Autodesk Fusion 360 part; units mm, degrees
sketch "Sketch1" plane through (0, 0, 0) normal (0, 1, 0) x (1, 0, 0)
  line L0 (125, 125) -> (-125, 125) construction
  line L1 (-125, 125) -> (-125, -125) construction
  line L2 (-125, -125) -> (125, -125) construction
  line L3 (125, -125) -> (125, 125) construction
  line L4 (125, 125) -> (-125, -125) construction
  line L5 (-125, 125) -> (125, -125) construction
  line L6 (75, 112.1152) -> (-75, 112.1152) construction
  line L7 (-75, 112.1152) -> (-75, 91.9152) construction
  line L8 (-75, 91.9152) -> (75, 91.9152) construction
  line L9 (75, 91.9152) -> (75, 112.1152) construction
  line L10 (75, 112.1152) -> (-75, 91.9152) construction
  line L11 (-75, 112.1152) -> (75, 91.9152) construction
  line L12 (137, 137) -> (92, 137)
  line L13 (92, 137) -> (137, 92)
  line L14 (137, 92) -> (137, 137)
  line L15 (125, 125) -> (137, 137) construction
  line L16 (128, 128) -> (109, 128) construction
  line L17 (109, 128) -> (128, 109) construction
  line L18 (128, 109) -> (128, 128) construction
  line L19 (92, 137) -> (84, 137)
  line L20 (84, 137) -> (84, 114)
  line L21 (84, 114) -> (104, 114)
  line L22 (104, 114) -> (114, 104)
  line L23 (114, 104) -> (114, 84)
  line L24 (114, 84) -> (137, 84)
  line L25 (137, 84) -> (137, 92)
  line L26 (84, 138) -> (-84, 138)
  line L27 (-84, 138) -> (-84, 113)
  line L28 (-84, 113) -> (84, 113)
  line L29 (84, 113) -> (84, 138)
  line L30 (84, 138) -> (-84, 113) construction
  line L31 (-84, 138) -> (84, 113) construction
  point P0 (0, 102.0152)
  point P1 (0, 125.5)
  dimension "d4" = 250
  dimension "d5" = 250
  dimension "d6" = 150
  dimension "d7" = 20.2
  dimension "d8" = 12
  dimension "d9" = 12
  dimension "d10" = 45
  dimension "d11" = 16
  dimension "d12" = 3
  dimension "d13" = 8
  dimension "d14" = 23
  dimension "d15" = 20
  dimension "d16" = 25
  dimension "d17" = 1
ref_plane "WorkPlane1" through (0, 7, 0) normal (0, 1, 0) x (0, 0, 1)
extrude "Extrude1" add sketch "Sketch1" along normal blind 4 contours L20 L26 L27 L28 L29
sketch "Sketch6" plane through (0, 4, 0) normal (0, 1, 0) x (-1, 0, 0)
  line L0 (-84, -113) -> (-84, -138)
  line L1 (-84, -138) -> (84, -138)
  line L2 (84, -138) -> (84, -113)
  line L3 (84, -113) -> (-84, -113)
  line L4 (-75, -135.575) -> (75, -135.575)
  line L5 (75, -135.575) -> (75, -115.425)
  line L6 (75, -115.425) -> (-75, -115.425)
  line L7 (-75, -115.425) -> (-75, -135.575)
  line L8 (-75, -135.575) -> (75, -115.425) construction
  line L9 (75, -135.575) -> (-75, -115.425) construction
  point P0 (0, -125.5)
  point P1 (0, -113)
  point P2 (84, -125.5)
  dimension "d36" = 150
  dimension "d37" = 20.15
extrude "Extrude4" add sketch "Sketch6" along normal up to surface (3 mm away) contours L4 L5 L6 L7
sketch "Sketch7" plane through (0, 4, 0) normal (0, 1, 0) x (-1, 0, 0)
  line L0 (75, -135.575) -> (-75, -135.575)
  line L1 (-75, -135.575) -> (-75, -115.425)
  line L2 (-75, -115.425) -> (75, -115.425)
  line L3 (75, -115.425) -> (75, -135.575)
  line L4 (-84, -113) -> (-84, -138)
  line L5 (-84, -138) -> (84, -138)
  line L6 (84, -138) -> (84, -113)
  line L7 (84, -113) -> (-84, -113)
  line L8 (-5, -135.575) -> (5, -135.575)
  line L9 (5, -135.575) -> (5, -138)
  line L10 (5, -138) -> (-5, -138)
  line L11 (-5, -138) -> (-5, -135.575)
  line L12 (-5, -135.575) -> (5, -138) construction
  line L13 (5, -135.575) -> (-5, -138) construction
  line L14 (-5, -113) -> (5, -113)
  line L15 (5, -113) -> (5, -115.425)
  line L16 (5, -115.425) -> (-5, -115.425)
  line L17 (-5, -115.425) -> (-5, -113)
  line L18 (-5, -113) -> (5, -115.425) construction
  line L19 (5, -113) -> (-5, -115.425) construction
  line L20 (-75, -135.575) -> (-65, -135.575)
  line L21 (-65, -135.575) -> (-65, -138)
  line L22 (-65, -138) -> (-75, -138)
  line L23 (-75, -138) -> (-75, -135.575)
  line L24 (-75, -115.425) -> (-65, -115.425)
  line L25 (-65, -115.425) -> (-65, -113)
  line L26 (-65, -113) -> (-75, -113)
  line L27 (-75, -113) -> (-75, -115.425)
  line L28 (75, -135.575) -> (65, -135.575)
  line L29 (65, -135.575) -> (65, -138)
  line L30 (65, -138) -> (75, -138)
  line L31 (75, -138) -> (75, -135.575)
  line L32 (75, -115.425) -> (65, -115.425)
  line L33 (65, -115.425) -> (65, -113)
  line L34 (65, -113) -> (75, -113)
  line L35 (75, -113) -> (75, -115.425)
  point P0 (0, -136.7875)
  point P1 (0, -114.2125)
  dimension "d42" = 10
extrude "Extrude5" add sketch "Sketch7" along normal blind 8 contours L0 L5 L28 L29 L30 L31 | L2 L7 L32 L33 L34 L35 | L0 L5 L8 L9 L10 L11 | L2 L7 L14 L15 L16 L17 | L0 L5 L20 L21 L22 L23 | L2 L7 L24 L25 L26 L27
chamfer "Chamfer1" distance 2 angle 45 12 edges at (-5, 12, -136.7875) (5, 12, -136.7875) (-5, 12, -114.2125) (5, 12, -114.2125) (-75, 12, -136.7875) (-65, 12, -136.7875) (-75, 12, -114.2125) (-65, 12, -114.2125) (65, 12, -136.7875) (75, 12, -136.7875) (65, 12, -114.2125) (75, 12, -114.2125)
sketch "Sketch9" plane through (0, 0, 0) normal (0, -1, 0) x (1, 0, 0)
  line L0 (84, -138) -> (84, -113)
  line L1 (84, -113) -> (-84, -113)
  line L2 (-84, -113) -> (-84, -138)
  line L3 (-84, -138) -> (84, -138)
  line L4 (84, -119.5) -> (90, -118)
  line L5 (90, -118) -> (90, -133)
  line L6 (90, -133) -> (84, -131.5)
  line L7 (90, -118) -> (84, -131.5) construction
  line L8 (90, -133) -> (84, -119.5) construction
  line L9 (90, -125.5) -> (84, -125.5) construction
  line L10 (84.0049, -119.5194) -> (89.98, -118.0256)
  line L11 (89.98, -118.0256) -> (89.98, -132.9744)
  line L12 (89.98, -132.9744) -> (84.0049, -131.4806)
  line L13 (84.0049, -131.4806) -> (84, -131.4794)
  line L14 (84.0049, -119.5194) -> (84, -119.5206)
  point P0 (90, -125.5)
  dimension "d51" = 12
  dimension "d52" = 15
  dimension "d53" = 6
  dimension "d56" = 0.02
extrude "Extrude7" add sketch "Sketch9" against normal blind 4 contours L0 L10 L11 L12 L13 L14
mirror "Mirror2" about plane through (0, 0, 0) normal (1, 0, 0) of "Extrude7"
fillet "Fillet2" radius 1 8 edges at (-84, 2, -119.5206) (-89.98, 2, -118.0256) (-84, 2, -131.4794) (-89.98, 2, -132.9744) (84, 2, -119.5206) (89.98, 2, -118.0256) (89.98, 2, -132.9744) (84, 2, -131.4794)
sketch "Sketch11" plane through (0, 7, 0) normal (0, 1, 0) x (-1, 0, 0)
  line L0 (-65, -115.425) -> (-75, -115.425)
  line L1 (-75, -115.425) -> (-75, -135.575)
  line L2 (-75, -135.575) -> (-65, -135.575)
  line L3 (-65, -135.575) -> (-5, -135.575)
  line L4 (-5, -135.575) -> (5, -135.575)
  line L5 (5, -135.575) -> (65, -135.575)
  line L6 (65, -135.575) -> (75, -135.575)
  line L7 (75, -135.575) -> (75, -115.425)
  line L8 (75, -115.425) -> (65, -115.425)
  line L9 (65, -115.425) -> (5, -115.425)
  line L10 (5, -115.425) -> (-5, -115.425)
  line L11 (-5, -115.425) -> (-65, -115.425)
  line L12 (65, -135.575) -> (5, -135.575)
  line L13 (5, -135.575) -> (5, -135.075)
  line L14 (5, -135.075) -> (65, -135.075)
  line L15 (65, -135.075) -> (65, -135.575)
  line L16 (65, -115.425) -> (5, -115.425)
  line L17 (5, -115.425) -> (5, -115.925)
  line L18 (5, -115.925) -> (65, -115.925)
  line L19 (65, -115.925) -> (65, -115.425)
  line L20 (-65, -135.575) -> (-5, -135.575)
  line L21 (-5, -135.575) -> (-5, -135.075)
  line L22 (-5, -135.075) -> (-65, -135.075)
  line L23 (-65, -135.075) -> (-65, -135.575)
  line L24 (-65, -115.425) -> (-5, -115.425)
  line L25 (-5, -115.425) -> (-5, -115.925)
  line L26 (-5, -115.925) -> (-65, -115.925)
  line L27 (-65, -115.925) -> (-65, -115.425)
  dimension "d63" = 0.5
extrude "Extrude8" cut sketch "Sketch11" against normal blind 3 contours L11 L24 L25 L26 L27 | L9 L16 L17 L18 L19 | L3 L20 L21 L22 L23 | L5 L12 L13 L14 L15
chamfer "Chamfer2" distance 2 angle 45 8 edges at (5, 4, -114.4625) (-5, 4, -114.4625) (-5, 4, -136.5375) (65, 4, -136.5375) (65, 4, -114.4625) (5, 4, -136.5375) (-65, 4, -114.4625) (-65, 4, -136.5375)
Check sheet for the modelled part. Datum: model origin and axes. Units: mm. A direction names the side the tool comes from. Give positions to 0.01 mm unless a question says otherwise; leave off trailing zeros. Order: outer loops, then holes, each group sorted by start corner. A loop starts at its lowest first (then second) coordinate and runs counter-clockwise, first axis right, second up. Notation, with made-up numbers: (76, 57.5) -> (88, 57.5) arc R25 cw to (88, 96.5) -> close; hole circle Ø6 at (5.25, 55). An arc over 180 degrees is marked (long way). Use CSV: the item, a comma, the result in double quotes. Start each with the question number.
1) Go/stop test with flat-tipped pins: P1, Ø1.5, axis at x = 35.5, z = -137, coming from the +Y side; P2, Ø1, axis at y = 6.5, z = -128, coming from the +X side; P3, Ø10, axis at x = -39, z = -130, coming from the +Y side; P4, Ø2, axis at y = 8.5, z = -130, coming from the -X side. Record where each tip stops, or that it passes through.
2) Sectioned sample at A-A, the plane x = 1. Record the boundary of the cut face in (y, z) (3 decimals).
3) Sectioned sample at B-B, the plane z = -129. Record the boundary of the cut face in (x, y).
4) Mould release check, pull along Z, two halves, no side actions. Record for faces 4 (the face through (-70, 9, -115.425)), 5 (the face through (-86.97, 1.97, -132.22)), 6 (the face through (84, 2, -135)): released by +Z, released by -Z, zero draft, split by the parting line, or undercut.
5) Sectioned sample at C-C, the plane x = 78. Record the boundary of the cut face in (y, z), plus the area to 3 significant figures.
6) Material ranges on line 1 (X direction, y = 7, z = -115); line 2 (X direction, y = 5.75, z = -113.75); line 3 (Y direction, x = 41, z = -131.25), recorded low to high. Write a range as from..to.
7) Set-up check for faces 1 (the face through (35, 4, -114)), 2 (the face through (35, 6, -135.075)), 3 (the face through (0, 9, -115.425)): record each of +Z, -Z, +X, -X, +Y, -Y from which the full face is reachable in a straight line by a thin tool's end or side.
Recorded:
1,P1,"y = 4"
1,P2,"x = 75"
1,P3,"y = 7"
1,P4,"through"
2,outline,"(0, -138) -> (12, -138) -> (12, -135.575) -> (7, -135.575) -> (7, -115.425) -> (12, -115.425) -> (12, -113) -> (0, -113) -> close"
3,outline,"(-89.98, 0) -> (89.98, 0) -> (89.98, 4) -> (75, 4) -> (75, 7) -> (-75, 7) -> (-75, 4) -> (-89.98, 4) -> close"
4,face 4,"undercut"
4,face 5,"released by -Z"
4,face 6,"zero draft"
5,outline,"(0, -138) -> (4, -138) -> (4, -113) -> (0, -113) -> close"
5,area,"100 mm2"
6,line 1,"-75..-65, -5..5, 65..75"
6,line 2,"-75..-64.75, -5.25..5.25, 64.75..75"
6,line 3,"0..7"
7,face 1,"+Z, +Y"
7,face 2,"-Z, +Y"
7,face 3,"+X, -X, +Y"
